```python
from build123d import *

# Parameters (mm, degrees)
SKETCH1_W           = 80
SKETCH1_H           = 50
BOSS_EXTRUDE1_DEPTH = 2.5
SKETCH2_W           = 80
SKETCH2_H           = 50
SKETCH2_W_2         = 76
SKETCH2_H_2         = 46
BOSS_EXTRUDE2_DEPTH = 20
SKETCH3_R           = 4
CUT_EXTRUDE1_DEPTH  = 20
SKETCH4_R           = 4
CUT_EXTRUDE2_DEPTH  = 20


with BuildPart() as part:
    # Sketch1 → Boss-Extrude1 (new body)
    with BuildSketch(Plane(origin=(0, 0, 0), x_dir=(1, 0, 0), z_dir=(0, 1, 0))):
        with Locations((40, -25)):
            Rectangle(SKETCH1_W, SKETCH1_H)
    extrude(amount=BOSS_EXTRUDE1_DEPTH)

    # Sketch2 → Boss-Extrude2 (add)
    with BuildSketch(Plane(origin=(0, 2.5, 0), x_dir=(1, 0, 0), z_dir=(0, 1, 0))):
        with Locations((40, -25)):
            Rectangle(SKETCH2_W, SKETCH2_H)
        with Locations((40, -25)):
            Rectangle(SKETCH2_W_2, SKETCH2_H_2, mode=Mode.SUBTRACT)
    extrude(amount=BOSS_EXTRUDE2_DEPTH)

    # Sketch3 → Cut-Extrude1 (cut)
    with BuildSketch(Plane.XY.offset(50)):
        with Locations((14.013555164, 12.601165946)):
            Circle(SKETCH3_R)
    extrude(amount=-CUT_EXTRUDE1_DEPTH, mode=Mode.SUBTRACT)

    # Sketch4 → Cut-Extrude2 (cut)
    with BuildSketch(Plane.XY.offset(2)):
        with Locations((59.449039137, 12.859939565)):
            Circle(SKETCH4_R)
    extrude(amount=-CUT_EXTRUDE2_DEPTH, mode=Mode.SUBTRACT)


solid = part.part
```
Verification items for the finished model (mm, model axes). A direction names the side the tool comes from. Coordinates: 2 decimals unless noted, no trailing zeros. Loops run counter-clockwise (first coordinate to the right, second up) from the corner with the lowest first, then second, coordinate; pieces in that order, holes last. Notation, with made-up numbers: (-38, 59.25) -> (13, 59.25) arc R25 cw to (13, 86.25) -> close; hole circle Ø9 at (16, -8). An arc over 180 degrees is marked (long way). Answer in a Markdown table with one row per item.
1) Section check C-C (y = 7). Record the cut outline in (x, z), and give its area (3 significant figures).
The answers:
| item | result |
|---|---|
| outline | (0, 0) -> (80, 0) -> (80, 50) -> (0, 50) -> close; hole (2, 2) -> (78, 2) -> (78, 48) -> (2, 48) -> close |
| area | 504 mm2 |
2) Depth check by flat-ended pin: P1, Ø10.5, axis at x = 14.01, y = 12.6, coming from the +Z side; P2, Ø14, axis at x = 50.5, z = 34.5, coming from the +Y side; P3, Ø5, axis at x = 59.45, y = 12.86, coming from the -Z side. Enter the tip coordinate at first touch or a pass-through.
The answers:
| item | result |
|---|---|
| P1 | stops at z = 50 |
| P2 | stops at y = 2.5 |
| P3 | stops at z = 48 |
3) Draft check along X on faces 1 (the face through (39, 12, 48)), 2 (the face through (80, 11, 25)), 3 (the face through (39, 0, 25)). Enter one of: released by +X, released by -X, zero draft, split by the parting line, or undercut.
The answers:
| item | result |
|---|---|
| face 1 | undercut |
| face 2 | released by +X |
| face 3 | zero draft |
4) Section check B-B (z = 12). Record the cut outline in (x, y).
The answers:
| item | result |
|---|---|
| outline | (0, 0) -> (80, 0) -> (80, 22.5) -> (78, 22.5) -> (78, 2.5) -> (2, 2.5) -> (2, 22.5) -> (0, 22.5) -> close |
5) Scan lines: line 1 along Z through (x, y) = (26, 9.25); line 2 along X through (y, z) = (18, 30); line 3 along Y through (x, z) = (16.5, 16). Record each from-to range of solid material in increasing order. Write a range as from..to.
The answers:
| item | result |
|---|---|
| line 1 | z = 0..2, 48..50 |
| line 2 | x = 0..2, 78..80 |
| line 3 | y = 0..2.5 |
6) Section check A-A (x = 54). Record the cut outline in (y, z), and give its area (3 significant figures).
The answers:
| item | result |
|---|---|
| outline | (0, 0) -> (22.5, 0) -> (22.5, 2) -> (2.5, 2) -> (2.5, 48) -> (22.5, 48) -> (22.5, 50) -> (0, 50) -> close |
| area | 205 mm2 |
7) Access from +Z, -Z, +X, -X, +Y, -Y to the whole of each face (thin tool, end or side, straight path). Record for faces 4 (the face through (39, 2.5, 25)), 5 (the face through (63.264, 14.061, 1.014)), 6 (the face through (10.839, 10.167, 49.014)), 7 (the face through (37, 22.5, 49)).
The answers:
| item | result |
|---|---|
| face 4 | +Y |
| face 5 | -Z |
| face 6 | +Z |
| face 7 | +Z, -Z, +X, -X, +Y |
8) Section check D-D (x = 13). Record the cut outline in (y, z), and give its area (3 significant figures).
The answers:
| item | result |
|---|---|
| outline | (0, 0) -> (22.5, 0) -> (22.5, 2) -> (2.5, 2) -> (2.5, 48) -> (8.73, 48) -> (8.73, 50) -> (0, 50) -> close; (16.47, 48) -> (22.5, 48) -> (22.5, 50) -> (16.47, 50) -> close |
| area | 190 mm2 |
